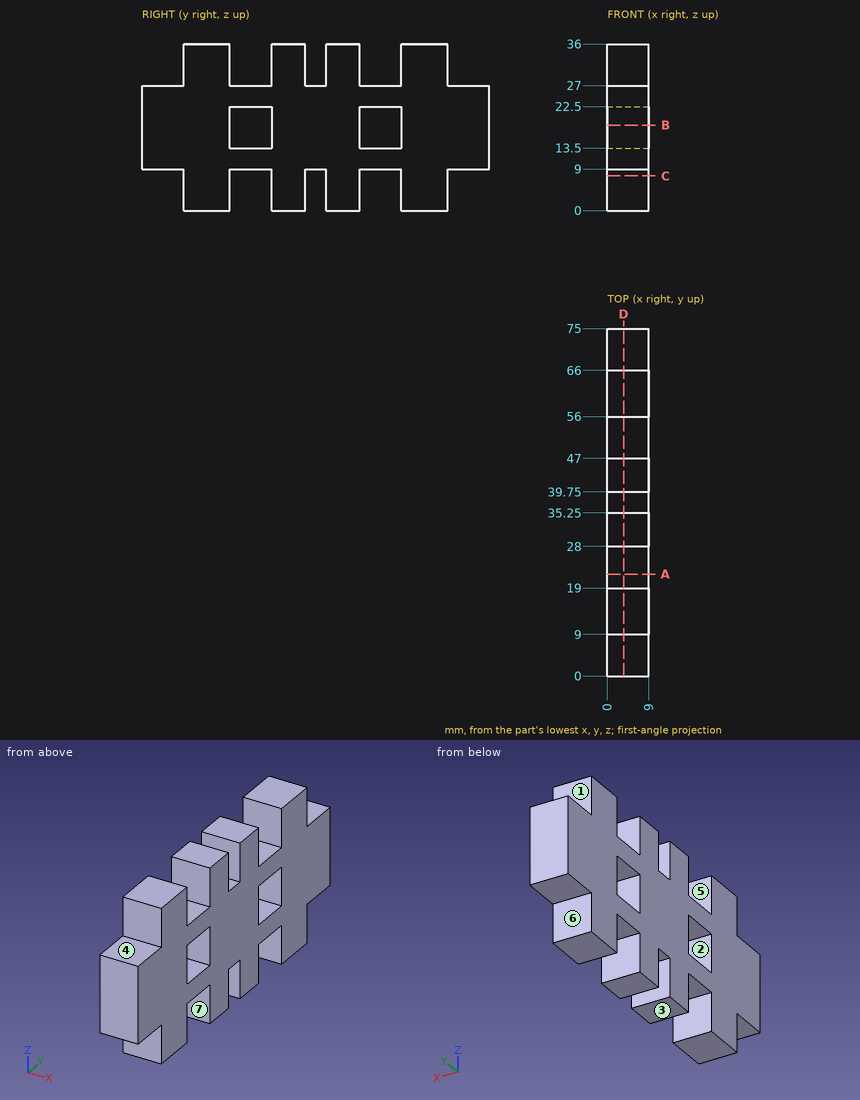
Here's the drawing with two shaded views (mm, measured from the low corner). I have some questions. A direction names the side the tool comes from. Round coordinates to 2 decimals unless told otherwise and drop trailing zeros. Order: outer loops, then holes, each group sorted by start corner. A loop starts at its lowest first (then second) coordinate and runs counter-clockwise, first axis right, second up. Notation, with made-up numbers: (70, -30.5) -> (120, -30.5) arc R13 cw to (120, -22.5) -> close; hole circle Ø1 at (69.25, -31). An arc over 180 degrees is marked (long way). Use a Markdown table: item, result. Add a question column.
(1) Suppose I cut it at C-C, the plane z = 7.5. Please give me the cut outline in (x, y), and give its area (4 significant figures).
(2) Suppose I cut it at D-D, the plane x = 3.5. Count the separate pieces of the cut face and the enclosed holes in it, and give its area (3 significant figures).
(3) Suppose I cut it at B-B, the plane z = 18.5. Please give me the cut outline in (x, y).
(4) If we mould it in two halves opening along Y, with no side actions, what happens to the marked faces 1, 2 and 3? For each: released by +Y, released by -Y, zero draft, split by the parting line, or undercut.
(5) I need wall thicknesses on line 1 along Y through (x, z) = (6, 29); line 2 along Y through (x, z) = (5.25, 14); line 3 along Z through (x, y) = (4.5, 25). Which ranges of each line are inside material? Lowest first, please.
(6) For the marked faces 4, 5, 6 and 7, which set-ups out of +Z, -Z, +X, -X, +Y, -Y let a thin tool reach every point of the face, with its end or its side?
(7) For pin 1 Ø4.5 at (x, z) = (6, 33) entering from +Y; pin 2 Ø2.5 at (x, y) = (3.5, 23.5) entering from -Z; pin 3 Ø4.5 at (x, y) = (4, 51.5) entering from +Z, each with a flat end and sliding along its axis, tell me the tip position at first contact or that it passes through.
(8) Suppose I cut it at A-A, the plane y = 22. Please give me the cut outline in (x, z), and give its area (3 significant figures).
Verdict:
| question | item | result |
|---|---|---|
| 1 | outline | (0, 9) -> (9, 9) -> (9, 19) -> (0, 19) -> close; (0, 28) -> (9, 28) -> (9, 35.25) -> (0, 35.25) -> close; (0, 39.75) -> (9, 39.75) -> (9, 47) -> (0, 47) -> close; (0, 56) -> (9, 56) -> (9, 66) -> (0, 66) -> close |
| 1 | area | 310.5 mm2 |
| 2 | separate pieces | 1 |
| 2 | enclosed holes | 2 |
| 2 | area | 1,810 mm2 |
| 3 | outline | (0, 0) -> (9, 0) -> (9, 19) -> (0, 19) -> close; (0, 28) -> (9, 28) -> (9, 47) -> (0, 47) -> close; (0, 56) -> (9, 56) -> (9, 75) -> (0, 75) -> close |
| 4 | face 1 | released by +Y |
| 4 | face 2 | undercut |
| 4 | face 3 | zero draft |
| 5 | line 1 | 9 to 19, 28 to 35.25, 39.75 to 47, 56 to 66 |
| 5 | line 2 | 0 to 19, 28 to 47, 56 to 75 |
| 5 | line 3 | 9 to 13.5, 22.5 to 27 |
| 6 | face 4 | +Z, +X, -X, -Y |
| 6 | face 5 | +Z, +X, -X |
| 6 | face 6 | -Z, +X, -X, +Y |
| 6 | face 7 | -Z, +X, -X |
| 7 | pin 1 | y = 66 |
| 7 | pin 2 | z = 9 |
| 7 | pin 3 | z = 27 |
| 8 | outline | (0, 9) -> (9, 9) -> (9, 13.5) -> (0, 13.5) -> close; (0, 22.5) -> (9, 22.5) -> (9, 27) -> (0, 27) -> close |
| 8 | area | 81.0 mm2 |
